Input: dimensioned drawing with shaded views. Units: mm. Origin: part minimum x, y, z. A direction names the side the tool comes from. Give positions to 0.01 mm unless a question says otherwise; leave off trailing zeros. Order: outer loops, then holes, each group sorted by start corner. A loop starts at its lowest first (then second) coordinate and runs counter-clockwise, first axis right, second up. Notation, with made-up numbers: M -31,71.5 L 23,71.5 A22 cw 23,88.5 Z; hole C 83,-4 d11. An arc over 180 degrees is marked long. Answer in a Markdown table with one row per item. Add a question column.
(1) Set-up query: the marked faces 1, 2 and 3. Return all of +Z, -Z, +X, -X, +Y, -Y with unobstructed straight access to the full face (end or side cutting, diameter ignored); none if empty.
(2) Section query B-B, the plane z = 9. Return loops of the section in (x, y).
(3) Section query A-A, the plane x = 51.25. Return loops of the section in (y, z).
(4) Section query D-D, the plane x = 17. Return loops of the section in (y, z), plus the area to 3 significant figures.
(5) Pin query (flat end, axial travel): P1, Ø1.5, axis at y = 13.5, z = 9.5, coming from the -X side; P2, Ø3, axis at y = 30.5, z = 12.5, coming from the +X side; P3, Ø5, axis at x = 24, z = 8.5, coming from the -Y side. Return the tip coordinate at first contact, or that it passes through.
(6) Material intervals for line 1 along X through (y, z) = (16.25, 13.75); line 2 along Z through (x, y) = (2, 15); line 3 along Y through (x, z) = (22, 11.5), sorted ascending.
(7) Section query C-C, the plane z = 14.25. Return loops of the section in (x, y), plus the area to 3 significant figures.
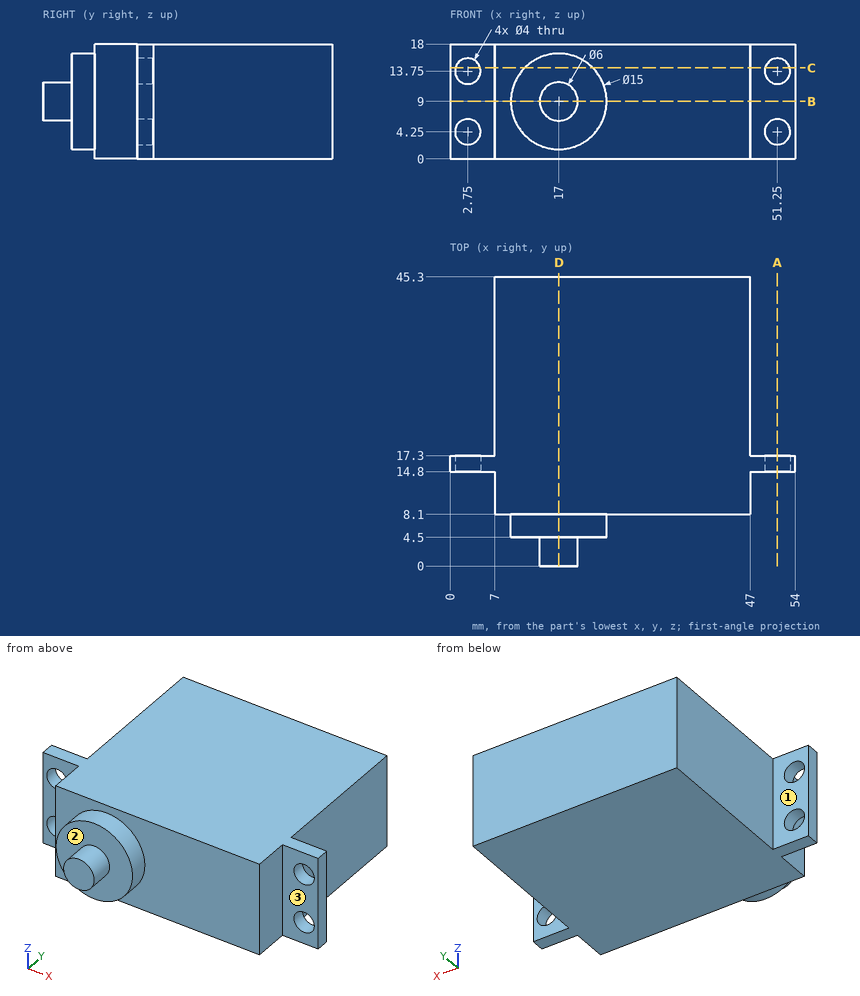
Values follow:
| question | item | result |
|---|---|---|
| 1 | face 1 | +Z, -Z, -X, +Y |
| 1 | face 2 | -Y |
| 1 | face 3 | +Z, -Z, +X, -Y |
| 2 | outline | M 0,14.8 L 7,14.8 L 7,8.1 L 9.5,8.1 L 9.5,4.5 L 14,4.5 L 14,0 L 20,0 L 20,4.5 L 24.5,4.5 L 24.5,8.1 L 47,8.1 L 47,14.8 L 54,14.8 L 54,17.3 L 47,17.3 L 47,45.3 L 7,45.3 L 7,17.3 L 0,17.3 Z |
| 3 | outline | M 14.8,0 L 17.3,0 L 17.3,2.25 L 14.8,2.25 Z; M 14.8,6.25 L 17.3,6.25 L 17.3,11.75 L 14.8,11.75 Z; M 14.8,15.75 L 17.3,15.75 L 17.3,18 L 14.8,18 Z |
| 4 | outline | M 0,6 L 4.5,6 L 4.5,1.5 L 8.1,1.5 L 8.1,0 L 45.3,0 L 45.3,18 L 8.1,18 L 8.1,16.5 L 4.5,16.5 L 4.5,12 L 0,12 Z |
| 4 | area | 751 mm² |
| 5 | P1 | stops at x = 7 |
| 5 | P2 | stops at x = 47 |
| 5 | P3 | stops at y = 4.5 |
| 6 | line 1 | x = 0 to 0.75, 4.75 to 49.25, 53.25 to 54 |
| 6 | line 2 | z = 0 to 2.4, 6.1 to 11.9, 15.6 to 18 |
| 6 | line 3 | y = 4.5 to 45.3 |
| 7 | outline | M 0,14.8 L 0.81,14.8 L 0.81,17.3 L 0,17.3 Z; M 4.69,14.8 L 7,14.8 L 7,8.1 L 11.64,8.1 L 11.64,4.5 L 22.36,4.5 L 22.36,8.1 L 47,8.1 L 47,14.8 L 49.31,14.8 L 49.31,17.3 L 47,17.3 L 47,45.3 L 7,45.3 L 7,17.3 L 4.69,17.3 Z; M 53.19,14.8 L 54,14.8 L 54,17.3 L 53.19,17.3 Z |
| 7 | area | 1,540 mm² |
